Can you work these out from the model? Positions are in its coordinate system, mm. Coordinates: 2 decimals unless noted, no trailing zeros. Write each loop counter-clockwise with the first axis right and the second up, starting at its lowest first coordinate (ties: lowest second). Pieces come first, ordered by that corner, then holes. Notation, with made-up numbers: (-38.5, -22.5) -> (15.5, -22.5) arc R19 ccw to (15.5, -3.5) -> close; hole circle Ø2 at (86, 18.5). An arc over 180 degrees is marked (long way). Use one line per item in the form item = value.
```python
from build123d import *

# Parameters (mm, degrees)
BOSS_EXTRUDE1_DEPTH = 6
CAVITY1_START       = -194.002075021
CAVITY1_DEPTH       = 186.04
CAVITY1_2_ANGLE     = 180
CAVITY1_3_ANGLE     = 180


with BuildPart() as part:
    # Sketch1 → Boss-Extrude1 (new body)
    with BuildSketch(Plane(origin=(0, -28.145825623, 0), x_dir=(1, 0, 0), z_dir=(0, 1, 0))):
        with BuildLine():
            Line((-10, 184.002075021), (-10, 17.962075021))
            ThreePointArc((-10, 17.962075021), (0, 7.962075021), (10, 17.962075021))
            Line((10, 17.962075021), (10, 184.002075021))
            ThreePointArc((10, 184.002075021), (0, 194.002075021), (-10, 184.002075021))
        make_face()
    extrude(amount=-BOSS_EXTRUDE1_DEPTH)

    # Cavity1: read off the stored shape, not the designer's step
    # Cavity1 outline → Cavity1 (cut)
    with BuildSketch(Plane.XY.offset(CAVITY1_START)):
        with BuildLine():
            Line((10, -34.145825623), (10, -31.145825623))
            ThreePointArc((10, -31.145825623), (9.121320344, -33.267145967), (7, -34.145825623))
            Line((7, -34.145825623), (10, -34.145825623))
        make_face()
        with BuildLine():
            Line((-10, -34.145825623), (-7, -34.145825623))
            ThreePointArc((-7, -34.145825623), (-9.121320344, -33.267145967), (-10, -31.145825623))
            Line((-10, -31.145825623), (-10, -34.145825623))
        make_face()
    extrude(amount=CAVITY1_DEPTH, mode=Mode.SUBTRACT)

    # Cavity1 2 outline → Cavity1 2 (revolve, cut)
    with BuildSketch(Plane.XY.offset(-184.002075021)):
        with BuildLine():
            ThreePointArc((10, -31.145825623), (9.121320344, -33.267145967), (7, -34.145825623))
            Line((7, -34.145825623), (10, -34.145825623))
            Line((10, -34.145825623), (10, -31.145825623))
        make_face()
    revolve(axis=Axis((0, 0, -184.002075021), (0, 1, 0)), revolution_arc=CAVITY1_2_ANGLE, mode=Mode.SUBTRACT)

    # Cavity1 3 outline → Cavity1 3 (revolve, cut)
    with BuildSketch(Plane(origin=(0, 0, -17.962075021), x_dir=(-1, 0, 0), z_dir=(0, 0, -1))):
        with BuildLine():
            ThreePointArc((10, -31.145825623), (9.121320344, -33.267145967), (7, -34.145825623))
            Line((7, -34.145825623), (10, -34.145825623))
            Line((10, -34.145825623), (10, -31.145825623))
        make_face()
    revolve(axis=Axis((0, 0, -17.962075021), (0, 1, 0)), revolution_arc=CAVITY1_3_ANGLE, mode=Mode.SUBTRACT)


solid = part.part
```
Q1. Suppose I cut it at A-A (z = -28). Write out the boundary of the cut face in (x, y).
Return value:
outline = (-10, -31.15) arc R3 ccw to (-7, -34.15) -> (7, -34.15) arc R3 ccw to (10, -31.15) -> (10, -28.15) -> (-10, -28.15) -> close
Q2. Will these pins go through, and if not, where does the flat tip stop? pin 1 (2 mm diameter, centred on x = -4, y = -30, fed in from +Z); pin 2 (2 mm diameter, centred on x = 3, y = -31.5, fed in from +Z).
Return value:
pin_1 = -8.42
pin_2 = -8.17
Q3. If I drill on line 1 (Z direction, x = 0.25, y = -29.3); line 2 (X direction, y = -31.25, z = -33); line 3 (Y direction, x = 8, z = -111.5), over which ranges is the centre line in solid material (lowest first)? Write a range as from..to.
Return value:
line_1 = -194..-7.97
line_2 = -10..10
line_3 = -33.97..-28.15
Q4. Suppose I cut it at B-B (y = -29.25). Write out the boundary of the cut face in (x, z).
Return value:
outline = (-10, -184) arc R10 ccw to (10, -184) -> (10, -17.96) arc R10 ccw to (-10, -17.96) -> close
